For this review, take the finished solid that the model builds, in its own axes (mm). A direction names the side the tool comes from. Round coordinates to 2 decimals unless told otherwise and drop trailing zeros. Write each loop counter-clockwise with the first axis right and the second up, starting at its lowest first coordinate (ties: lowest second). Pieces come first, ordered by that corner, then holes.
Autodesk Fusion 360 part; units mm, degrees
sketch "Sketch1" plane through (0, 0, 0) normal (0, 0, 1) x (1, 0, 0)
  line L0 (0, 0) -> (70, 0)
  line L1 (70, 0) -> (70, 20)
  line L2 (70, 20) -> (0, 20)
  line L3 (0, 20) -> (0, 0)
  line L4 (35, 0) -> (35, 2)
  line L5 (35, 2) -> (5, 2)
  line L6 (5, 2) -> (5, 20)
  line L7 (65, 2) -> (65, 20)
  line L8 (35, 2) -> (65, 2)
  line L9 (5, 2) -> (5, 0)
  line L10 (65, 2) -> (65, 0)
  dimension "d2" = 70
  dimension "d3" = 20
  dimension "d5" = 2
  dimension "d6" = 30
extrude "Extrude1" add sketch "Sketch1" along normal blind 3 contours L0 L2 L3 L6 L9 | L0 L4 L5 L9 | L0 L4 L8 L10 | L0 L1 L2 L7 L10
chamfer "Chamfer1" distance 4 distance2 4 1 edges at (65, 20, 1.5) measured on face at (68.3333, 20, 1)
chamfer "Chamfer1" distance 4 distance2 4 1 edges at (5, 20, 1.5) measured on face at (5, 8, 1)
fillet "Fillet1" radius 1 4 edges at (5, 16, 1.5) (1, 20, 1.5) (65, 16, 1.5) (69, 20, 1.5)
fillet "Fillet2" radius 0.5 9 edges at (35, 2, 3) (69.0315, 19.9239, 3) (67, 18, 3) (65.0761, 15.9685, 3) (65, 8.7929, 3) (5, 8.7929, 3) (4.9239, 15.9685, 3) (3, 18, 3) (0.9685, 19.9239, 3)
extrude "Extrude2" add sketch "Sketch1" along normal blind 10 contours L0 L4 L5 L9 | L0 L4 L8 L10
equation "box_width = 70 mm"
equation "d2 = box_width"
equation "d3 = box_len"
equation "cover_width = 60 mm"
equation "d6 = cover_width / 2"
equation "box_len = 20 mm"
(1) For pin 1 Ø1 at (y, z) = (1, 8) entering from -X; pin 2 Ø8 at (x, y) = (19, 7.5) entering from -Z; pin 3 Ø2 at (y, z) = (7.5, 1) entering from -X; pin 4 Ø1.5 at (x, y) = (68, 13) entering from +Z, all flat-tipped, find the tip position at first contact; note any pin that passes through.
Geometry check:
pin 1: stops at x = 5
pin 2: passes through
pin 3: stops at x = 0
pin 4: stops at z = 3
(2) For line 1 along X through (y, z) = (7, 2.5); line 2 along Z through (x, y) = (66, 14.75); line 3 along Y through (x, z) = (57.5, 2.5), list the stretches that pass through material, from the lowest coordinate up.
Geometry check:
line 1: x = 0 to 5, 65 to 70
line 2: z = 0 to 3
line 3: y = 0 to 2
(3) For faces 4 (the face through (2.87, 17.918, 2.857)), 5 (the face through (35, 2, 5)), 6 (the face through (35, 1, 0)), 7 (the face through (68, 10, 3)), list the 3-axis set-ups (+Z, -Z, +X, -X, +Y, -Y) from which the entire face can be reached by the end or side of a thin tool; tool diameter is ignored.
Geometry check:
face 4: +Z, +Y
face 5: +Z, -Z, +Y
face 6: -Z, +X, -X, +Y, -Y
face 7: +Z, +X, +Y, -Y
(4) Mouldability with a two-part tool opening along X and no side actions: class faces 1 (the face through (0, 10, 1)), 2 (the face through (35, 1, 10)), 3 (the face through (65, 9, 1)) as pulls with the +X half, pulls with the -X half, needs draft (parallel to the pull), parting line crosses it, or undercut.
Geometry check:
face 1: pulls with the -X half
face 2: needs draft
face 3: undercut
(5) We need section C-C, the plane z = 7. Give the boundary of the cut face in (x, y), and give its area (3 significant figures).
Geometry check:
outline: (5, 0) - (65, 0) - (65, 2) - (5, 2) - close
area: 120 mm2
(6) We need section B-B, the plane x = 29. Give the boundary of the cut face in (y, z), and give its area (3 significant figures).
Geometry check:
outline: (0, 0) - (2, 0) - (2, 10) - (0, 10) - close
area: 20.0 mm2
(7) We need section A-A, the plane y = 8.5. Give the boundary of the cut face in (x, z), and give its area (3 significant figures).
Geometry check:
outline: (0, 0) - (5, 0) - (5, 2.5) arc R0.5 ccw to (4.5, 3) - (0, 3) - close; (65, 0) - (70, 0) - (70, 3) - (65.5, 3) arc R0.5 ccw to (65, 2.5) - close
area: 29.9 mm2
